Read the model definition and answer for the solid it produces. Units are mm, in the model's axes. A direction names the side the tool comes from. Coordinates: 2 decimals unless noted, no trailing zeros. Loops run counter-clockwise (first coordinate to the right, second up) from the corner with the lowest first, then second, coordinate; pieces in that order, holes last.
Q1. Flat-ended cylindrical pins translate along their axes: P1, Ø8.5, axis at x = -31.5, z = 0, coming from the -Y side; P2, Ø1, axis at x = -42, y = -10, coming from the -Z side; P3, Ø8.5, axis at x = -51.5, z = 0, coming from the +Y side; P4, Ø5, axis at x = -52, y = -3.5, coming from the -Z side. Find the tip coordinate at first contact, or state that the pin passes through.
Q2. Section C-C (x = -59) is taken. Give the vertices of the cut face in (y, z).
Q3. The mould has two halves that part along X. Classify faces 1 (the face through (-63.007, -21.199, -11.215)), 2 (the face through (-61.5, -11, -1)), 3 (the face through (-48.9, 0, 0.1)): pulls with the +X half, pulls with the -X half, needs draft (parallel to the pull), parting line crosses it, or undercut.
Q4. Section A-A (z = 0) is taken. Give the vertices of the cut face in (x, y), then the cut area to 3 significant figures.
Q5. Section B-B (x = -51.5) is taken. Give the vertices of the cut face in (y, z).
Q6. Which of the six approach directions +Z, -Z, +X, -X, +Y, -Y give full straight-line access (tool end or side, diameter ignored) to faces 4 (the face through (-61.215, -11.626, 8.199)), 5 (the face through (-21.5, 0, 2))?
Q7. Straight lines are drawn through the part: line 1 (X direction, y = -6, z = 2); line 2 (Y direction, x = -37, z = 4.5); line 3 (Z direction, x = -51.5, y = -0.5). For each, find the intervals that lie inside material, in ascending order.
from build123d import *

# Parameters (mm, degrees)
F0_W     = 43
F0_H     = 23
F0_R     = 2.6
F1_DEPTH = 1.5
F3_DEPTH = 20
F5_DEPTH = 3.001
F7_DEPTH = 3.001
F8_R     = 1


with BuildPart() as f1:
    # F0 (on Front) → F1 (new body, symmetric)
    with BuildSketch(Plane.XZ):
        Rectangle(F0_W, F0_H)
        with Locations((-11.5, 0)):
            Circle(F0_R, mode=Mode.SUBTRACT)
        with Locations((8.5, 0)):
            Circle(F0_R, mode=Mode.SUBTRACT)
    extrude(amount=F1_DEPTH, both=True)

    # F2 (on face) → F3 (join)
    with BuildSketch(Plane.XZ.offset(1.5)):
        Polygon((21.5, -11.5), (21.5, 11.5), (-21.5, 11.5), (-21.5, 8.5), (18.5, 8.5), (18.5, -11.5), align=None)
    extrude(amount=F3_DEPTH)

    # F4 (on face) → F5 (cut, through all)
    with BuildSketch(Plane(origin=(0, 0, 8.5), x_dir=(1, 0, 0), z_dir=(0, 0, -1))):
        with BuildLine():
            ThreePointArc((9.1542480146, 14.0163385176), (5.9836614824, 12.1542480146), (7.8457519854, 8.9836614824))
            Line((7.8457519854, 8.9836614824), (9.1542480146, 14.0163385176))
        make_face()
        with BuildLine():
            Line((9.1542480146, 14.0163385176), (7.8457519854, 8.9836614824))
            ThreePointArc((7.8457519854, 8.9836614824), (10.0904331426, 9.4431766194), (11.1, 11.5))
            ThreePointArc((11.1, 11.5), (10.5568233806, 13.0904331426), (9.1542480146, 14.0163385176))
        make_face()
    extrude(amount=-F5_DEPTH, mode=Mode.SUBTRACT)

    # F6 (on face) → F7 (cut, through all)
    with BuildSketch(Plane(origin=(0, 0, 8.5), x_dir=(1, 0, 0), z_dir=(0, 0, -1))):
        Polygon((-21.5, 3.5), (3.5, 21.5), (-21.5, 21.5), align=None)
    extrude(amount=-F7_DEPTH, mode=Mode.SUBTRACT)

    # F8
    f8_edges = [f1.edges().sort_by_distance(p)[0] for p in [
        (21.5, 1.5, 0),
        (21.5, -10, 11.5),
        (21.5, -21.5, 0),
        (21.5, -10, -11.5),
        (0, 1.5, -11.5),
        (0, 1.5, 11.5),
        (-21.5, -1, 11.5),
        (-9, -12.5, 11.5),
        (12.5, -21.5, 11.5),
        (-9, -12.5, 8.5),
        (3.5, -21.5, 10),
        (11, -21.5, 8.5),
        (18.5, -21.5, -1.5),
        (-1.5, -1.5, -11.5),
        (18.5, -11.5, 8.5),
        (18.5, -11.5, -11.5),
        (18.5, -1.5, -1.5),
        (20, -21.5, -11.5),
        (-21.5, 0, -11.5),
        (-21.5, 1.5, 0),
        (-21.5, -1.5, -1.5),
        (-21.5, -2.5, 8.5),
        (-21.5, -3.5, 10),
        (-1.5, -1.5, 8.5),
    ]]
    fillet(f8_edges, radius=F8_R)


with BuildPart() as f10_1:
    # F10: instance of F1
    add(f1.part.mirror(Plane(origin=(-21.5, -0.2115756963, 1.3410341816), x_dir=(0, -1, 0), z_dir=(-1, 0, 0))))


solid = f10_1.part
Numbers:
1. P1: stops at y = -1.5
1. P2: stops at z = 8.5
1. P3: stops at y = 1.5
1. P4: stops at z = -11.37
2. outline: (-21.5, 9.5) arc R1 ccw to (-20.5, 8.5) - (-2.5, 8.5) arc R1 cw to (-1.5, 7.5) - (-1.5, -10.5) arc R1 ccw to (-0.5, -11.5) - (0.5, -11.5) arc R1 ccw to (1.5, -10.5) - (1.5, 10.5) arc R1 ccw to (0.5, 11.5) - (-20.5, 11.5) arc R1 ccw to (-21.5, 10.5) - close
3. face 1: needs draft
3. face 2: pulls with the +X half
3. face 3: undercut
4. outline: (-64.5, -20.5) arc R1 ccw to (-63.5, -21.5) - (-62.5, -21.5) arc R1 ccw to (-61.5, -20.5) - (-61.5, -2.5) arc R1 cw to (-60.5, -1.5) - (-54.1, -1.5) - (-54.1, 1.5) - (-63.5, 1.5) arc R1 ccw to (-64.5, 0.5) - close; (-48.9, -1.5) - (-34.1, -1.5) - (-34.1, 1.5) - (-48.9, 1.5) - close; (-28.9, -1.5) - (-22.5, -1.5) arc R1 ccw to (-21.5, -0.5) - (-21.5, 0.5) arc R1 ccw to (-22.5, 1.5) - (-28.9, 1.5) - close
4. area: 157 mm2
5. outline: (-21.5, 9.5) arc R1 ccw to (-20.5, 8.5) - (-14.1, 8.5) - (-14.1, 11.5) - (-20.5, 11.5) arc R1 ccw to (-21.5, 10.5) - close; (-8.9, 8.5) - (-2.5, 8.5) arc R1 cw to (-1.5, 7.5) - (-1.5, 2.6) - (1.5, 2.6) - (1.5, 10.5) arc R1 ccw to (0.5, 11.5) - (-8.9, 11.5) - close; (-1.5, -10.5) arc R1 ccw to (-0.5, -11.5) - (0.5, -11.5) arc R1 ccw to (1.5, -10.5) - (1.5, -2.6) - (-1.5, -2.6) - close
6. face 4: -Z, +X, -Y
6. face 5: +Z, -Z, +X, +Y, -Y
7. line 1: x = -64.5 to -61.5
7. line 2: y = -1.5 to 1.5
7. line 3: z = -11.5 to -2.6, 2.6 to 11.5
